Could you check a few things on this drawing? It's one solid part, dimensions in mm from its lowest x, y, z. Round coordinates to 2 decimals unless told otherwise and drop trailing zeros. Loops run counter-clockwise (first coordinate to the right, second up) from the corner with the lowest first, then second, coordinate; pieces in that order, holes last. Notation, with made-up numbers: (10.25, -18) -> (27.25, -18) arc R25 cw to (27.25, 6) -> close; hole circle Ø5 at (53, 65). An arc over 180 degrees is marked (long way). Write each question's results on one line, items separated by ' | '.
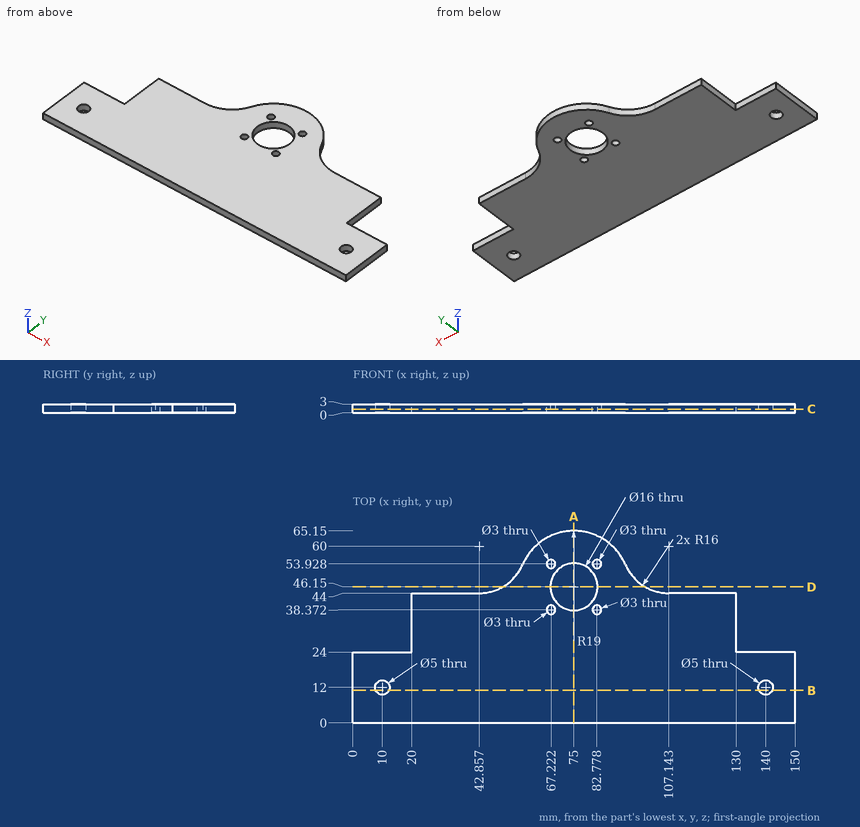
1) I want a section at B-B, the plane y = 11. Write out the boundary of the cut face in (x, z).
Model answer:
outline: (0, 0) -> (7.71, 0) -> (7.71, 3) -> (0, 3) -> close; (12.29, 0) -> (137.71, 0) -> (137.71, 3) -> (12.29, 3) -> close; (142.29, 0) -> (150, 0) -> (150, 3) -> (142.29, 3) -> close
2) I need wall thicknesses on line 1 (X direction, y = 12, z = 1); line 2 (Y direction, x = 140, z = 1.75); line 3 (X direction, y = 11, z = 1.8). Which ranges of each line are inside material? Lowest first, please.
Model answer:
line 1: x = 0 to 7.5, 12.5 to 137.5, 142.5 to 150 | line 2: y = 0 to 9.5, 14.5 to 24 | line 3: x = 0 to 7.71, 12.29 to 137.71, 142.29 to 150
3) I want a section at A-A, the plane x = 75. Write out the boundary of the cut face in (y, z).
Model answer:
outline: (0, 0) -> (38.15, 0) -> (38.15, 3) -> (0, 3) -> close; (54.15, 0) -> (65.15, 0) -> (65.15, 3) -> (54.15, 3) -> close
4) I want a section at D-D, the plane y = 46.15. Write out the boundary of the cut face in (x, z).
Model answer:
outline: (50.87, 0) -> (67, 0) -> (67, 3) -> (50.87, 3) -> close; (83, 0) -> (99.13, 0) -> (99.13, 3) -> (83, 3) -> close
5) I'm going to push flat-ended pins straight in: pin 1 (0.9 mm diameter, centred on x = 28.5, z = 2, fed in from +Y); pin 2 (0.9 mm diameter, centred on x = 11, z = 1.5, fed in from +Y); pin 3 (0.9 mm diameter, centred on y = 32.5, z = 2, fed in from -X). Where does each tip first touch, or does it pass through?
Model answer:
pin 1: stops at y = 44 | pin 2: stops at y = 24 | pin 3: stops at x = 20
6) I want a section at C-C, the plane z = 1.25. Write out the boundary of the cut face in (x, y), plus the area to 3 significant figures.
Model answer:
outline: (0, 0) -> (150, 0) -> (150, 24) -> (130, 24) -> (130, 44) -> (107.14, 44) arc R16 cw to (92.45, 53.67) arc R19 ccw to (57.55, 53.67) arc R16 cw to (42.86, 44) -> (20, 44) -> (20, 24) -> (0, 24) -> close; hole circle Ø5 at (10, 12); hole circle Ø3 at (67.22, 38.37); hole circle Ø3 at (67.22, 53.93); hole circle Ø16 at (75, 46.15); hole circle Ø3 at (82.78, 38.37); hole circle Ø3 at (82.78, 53.93); hole circle Ø5 at (140, 12) | area: 6,240 mm2
